from build123d import *

# Parameters (mm, degrees)
BOSS_EXTRUDE1_DEPTH = 18
BOSS_EXTRUDE2_DEPTH = 9
CUT_EXTRUDE1_DEPTH  = 28
SKETCH3_R           = 25
SKETCH3_R_2         = 18
BOSS_EXTRUDE3_DEPTH = 22
SKETCH3_2_R         = 18
CUT_EXTRUDE2_DEPTH  = 41
SKETCH6_R           = 4
BOSS_EXTRUDE5_DEPTH = 10
SKETCH7_W           = 57.081853501
SKETCH7_H           = 4
CUT_EXTRUDE3_DEPTH  = 40


with BuildPart() as part:
    # Sketch1 → Boss-Extrude1 (new body)
    with BuildSketch(Plane.XY):
        with BuildLine():
            Line((110, 12), (2.973910519, 24.822486906))
            ThreePointArc((2.973910519, 24.822486906), (-25, 0), (2.973910519, -24.822486906))
            Line((2.973910519, -24.822486906), (110, -12))
            ThreePointArc((110, -12), (122, 0), (110, 12))
        make_face()
    extrude(amount=-BOSS_EXTRUDE1_DEPTH)

    # Sketch2 → Boss-Extrude2 (add)
    with BuildSketch(Plane.XY.offset(9)):
        with BuildLine():
            Line((110, -12), (70, -12))
            ThreePointArc((70, -12), (58, 0), (70, 12))
            Line((70, 12), (110, 12))
            ThreePointArc((110, 12), (122, 0), (110, -12))
        make_face()
        with BuildLine():
            Line((70, 6), (110, 6))
            ThreePointArc((110, 6), (116, 0), (110, -6))
            Line((110, -6), (70, -6))
            ThreePointArc((70, -6), (64, 0), (70, 6))
        make_face(mode=Mode.SUBTRACT)
    extrude(amount=-BOSS_EXTRUDE2_DEPTH)

    # Sketch2<2> → Cut-Extrude1 (cut, through all)
    with BuildSketch(Plane.XY.offset(9)):
        with BuildLine():
            Line((70, -6), (110, -6))
            ThreePointArc((110, -6), (116, 0), (110, 6))
            Line((110, 6), (70, 6))
            ThreePointArc((70, 6), (64, 0), (70, -6))
        make_face()
    extrude(amount=-CUT_EXTRUDE1_DEPTH, mode=Mode.SUBTRACT)

    # Sketch3 → Boss-Extrude3 (add)
    with BuildSketch(Plane.XY.offset(22)):
        Circle(SKETCH3_R)
        Circle(SKETCH3_R_2, mode=Mode.SUBTRACT)
    extrude(amount=-BOSS_EXTRUDE3_DEPTH)

    # Sketch3<2> → Cut-Extrude2 (cut, through all)
    with BuildSketch(Plane.XY.offset(22)):
        Circle(SKETCH3_2_R)
    extrude(amount=-CUT_EXTRUDE2_DEPTH, mode=Mode.SUBTRACT)

    # Sketch6 → Boss-Extrude5 (add, symmetric)
    with BuildSketch(Plane(origin=(0, 0, 0), x_dir=(1, 0, 0), z_dir=(0, 1, 0))):
        with BuildLine():
            Line((-19, 12), (-32, 12))
            ThreePointArc((-32, 12), (-42, 2), (-32, -8))
            Line((-32, -8), (-19, -8))
            Line((-19, -8), (-19, 12))
        make_face()
        with Locations((-32, 2)):
            Circle(SKETCH6_R, mode=Mode.SUBTRACT)
    extrude(amount=BOSS_EXTRUDE5_DEPTH, both=True)

    # Sketch7 → Cut-Extrude3 (cut)
    with BuildSketch(Plane(origin=(-42, 0, 0), x_dir=(0, 0, -1), z_dir=(1, 0, 0))):
        with Locations((1.514511954, 0)):
            Rectangle(SKETCH7_W, SKETCH7_H)
    extrude(amount=CUT_EXTRUDE3_DEPTH, mode=Mode.SUBTRACT)


solid = part.part
Could you check a few things on this model? Use its own coordinates, in mm. A direction names the side the tool comes from. Coordinates: 2 decimals unless noted, no trailing zeros. Loops run counter-clockwise (first coordinate to the right, second up) from the corner with the lowest first, then second, coordinate; pieces in that order, holes last.
1. We'd pull the mould along Y, two halves only. Please class faces 1 (the face through (-35.2, -6.1, 0.4)), 2 (the face through (-27, -2, 2)), 3 (the face through (90, -12, 5)): released by +Y, released by -Y, zero draft, split by the parting line, or undercut.
2. I need wall thicknesses on L1, parallel to Z at x = -32, y = -4; L2, parallel to X at y = 6.5, z = 4; L3, parallel to X at y = 0, z = -2.5. Which ranges of each line are inside material? Lowest first, please.
3. Imagine slicing it at A-A (z = -2). Please give me the cut outline in (x, y).
4. Imagine slicing it at C-C (y = -8). Please give me the cut outline in (x, z).
5. For P1, Ø1.5, axis at x = 87.5, z = 3, coming from the +Y side; P2, Ø10, axis at y = -1, z = 15.5, coming from the -X side; P3, Ø6, axis at x = -10, z = -6.5, coming from the -Y side, each with a flat end and sliding along its axis, tell me the tip position at first contact or that it passes through.
6. Imagine slicing it at B-B (y = 4). Please give me the cut outline in (x, z), and give its area (3 significant figures).
7. For faces 4 (the face through (90, 12, 5)), 5 (the face through (-27, 2, 2)), 6 (the face through (44, -2, 0)), 7 (the face through (-28, 10, 0)), 8 (the face through (116, 0, -4)), which set-ups out of +Z, -Z, +X, -X, +Y, -Y let a thin tool reach every point of the face, with its end or its side?
8. Imagine slicing it at D-D (z = -9). Please give me the cut outline in (x, y), and give its area (3 significant figures).
Computed values:
1. face 1: zero draft
1. face 2: undercut
1. face 3: released by -Y
2. L1: z = -12 to -6, 2 to 8
2. L2: x = -40 to -16.79, 16.79 to 24.14, 59.91 to 120.09
2. L3: x = 18 to 64, 116 to 122
3. outline: (-42, -10) - (-36, -10) - (-36, -2) - (-42, -2) - close; (-42, 2) - (-36, 2) - (-36, 10) - (-42, 10) - close; (-28, -10) - (-22.91, -10) arc R25 ccw to (2.97, -24.82) - (110, -12) arc R12 ccw to (110, 12) - (2.97, 24.82) arc R25 ccw to (-22.91, 10) - (-28, 10) - (-28, 2) - (-17.89, 2) arc R18 cw (long way) to (-17.89, -2) - (-28, -2) - close; hole (70, -6) - (110, -6) arc R6 ccw to (110, 6) - (70, 6) arc R6 ccw to start
4. outline: (-32, -12) - (-23.69, -12) - (-23.69, -18) - (-16.12, -18) - (-16.12, 22) - (-23.69, 22) - (-23.69, 8) - (-32, 8) arc R10 ccw to start; (16.12, -18) - (118.94, -18) - (118.94, 9) - (61.06, 9) - (61.06, 0) - (23.69, 0) - (23.69, 22) - (16.12, 22) - close; hole circle Ø8 at (-32, -2)
5. P1: stops at y = 12
5. P2: stops at x = -24.92
5. P3: stops at y = -24
6. outline: (-32, -12) - (-24.68, -12) - (-24.68, -18) - (-17.55, -18) - (-17.55, 22) - (-24.68, 22) - (-24.68, 8) - (-32, 8) arc R10 ccw to start; (17.55, -18) - (65.53, -18) - (65.53, 9) - (58.69, 9) - (58.69, 0) - (24.68, 0) - (24.68, 22) - (17.55, 22) - close; (114.47, -18) - (121.31, -18) - (121.31, 9) - (114.47, 9) - close; hole circle Ø8 at (-32, -2)
6. area: 1,810 mm2
7. face 4: +Z, +X, +Y
7. face 5: +Z, -Z, -X
7. face 6: +Z
7. face 7: +Z, -Z, -X, +Y
7. face 8: +Z, -Z
8. outline: (-39.14, -10) - (-22.91, -10) arc R25 ccw to (2.97, -24.82) - (110, -12) arc R12 ccw to (110, 12) - (2.97, 24.82) arc R25 ccw to (-22.91, 10) - (-39.14, 10) - (-39.14, 2) - (-17.89, 2) arc R18 cw (long way) to (-17.89, -2) - (-39.14, -2) - close; hole (70, -6) - (110, -6) arc R6 ccw to (110, 6) - (70, 6) arc R6 ccw to start
8. area: 3,900 mm2
